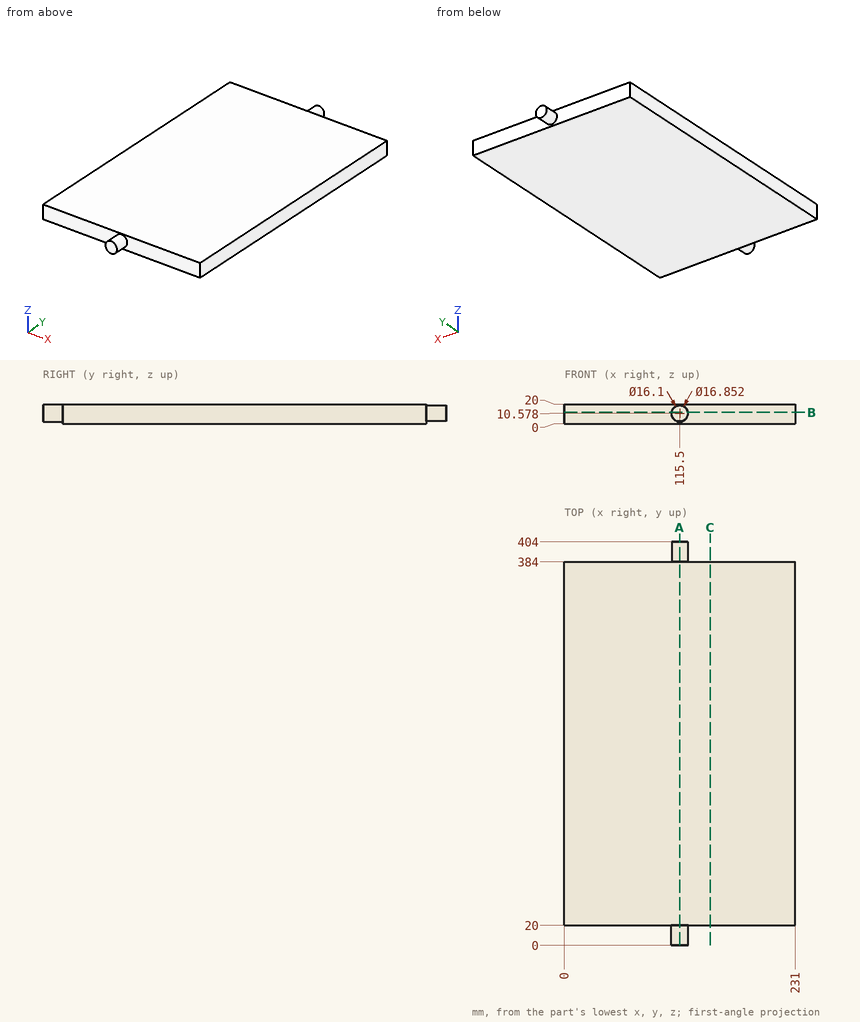
Could you check a few things on this drawing? It's one solid part, dimensions in mm from its lowest x, y, z. Round coordinates to 2 decimals unless told otherwise and drop trailing zeros. Order: outer loops, then holes, each group sorted by start corner. A loop starts at its lowest first (then second) coordinate and runs counter-clockwise, first axis right, second up. Notation, with made-up numbers: M -27,-18 L -23,-18 A26 ccw -23,9 Z; hole C 89,-31 d4. An arc over 180 degrees is marked long. One line per item, written item: value.
(1) I'm going to push flat-ended pins straight in: P1, Ø6, axis at x = 98.5, z = 10.5, coming from the +Y side; P2, Ø6, axis at x = 59, z = 7.5, coming from the -Y side. Where does each tip first touch, or does it pass through?
Ans:
P1: stops at y = 384
P2: stops at y = 20
(2) Imagine slicing it at B-B (z = 11.5). Write out the boundary of the cut face in (x, y) (1 decimal), and give its area (3 significant figures).
Ans:
outline: M 0,20 L 107.1,20 L 107.1,0 L 123.9,0 L 123.9,20 L 231,20 L 231,384 L 123.5,384 L 123.5,404 L 107.5,404 L 107.5,384 L 0,384 Z
area: 84,700 mm^2
(3) I need wall thicknesses on line 1 along Y through (x, z) = (95, 7.5); line 2 along Y through (x, z) = (121.5, 5). Which ranges of each line are inside material? Lowest first, please. Write a range as from..to.
Ans:
line 1: y = 20..384
line 2: y = 0..384
(4) Imagine slicing it at A-A (x = 115.5). Write out the boundary of the cut face in (y, z), and give its area (3 significant figures).
Ans:
outline: M 0,2.15 L 20,2.15 L 20,0 L 384,0 L 384,2.53 L 404,2.53 L 404,18.63 L 384,18.63 L 384,20 L 20,20 L 20,19 L 0,19 Z
area: 7,940 mm^2
(5) Imagine slicing it at C-C (x = 146). Write out the boundary of the cut face in (y, z).
Ans:
outline: M 20,0 L 384,0 L 384,20 L 20,20 Z
